from build123d import *

# Parameters (mm, degrees)
BOSS_EXTRUDE1_DEPTH = 17
BOSS_EXTRUDE2_DEPTH = 1.5
SKETCH3_R           = 1.45
CUT_EXTRUDE1_DEPTH  = 45.735332792
FILLET1_R           = 10
SKETCH4_R           = 5
CUT_EXTRUDE4_DEPTH  = 2
FILLET2_R           = 0.5
SKETCH5_W           = 31
SKETCH5_H           = 3
BOSS_EXTRUDE3_DEPTH = 30
SKETCH6_W           = 3
SKETCH6_H           = 3
BOSS_EXTRUDE4_DEPTH = 10
CHAMFER1_SIZE2      = 10
CHAMFER1_SIZE       = 2.679491924
FILLET3_R           = 5
FILLET4_R           = 2


# Some blends are built 0.0001 mm under size
with BuildPart() as part:
    # Sketch1 → Boss-Extrude1 (new, symmetric)
    with BuildSketch(Plane(origin=(0, 0, 0), x_dir=(1, 0, 0), z_dir=(0, 1, 0))):
        Polygon((15.5, 0), (-15.5, 0), (-15.5, 30), (-18.5, 30), (-18.5, -3), (-28.5, -3), (-28.5, -6), (28.5, -6), (28.5, -3), (18.5, -3), (18.5, 30), (15.5, 30), align=None)
    extrude(amount=BOSS_EXTRUDE1_DEPTH, both=True)

    # Sketch2 → Boss-Extrude2 (add, symmetric)
    with BuildSketch(Plane(origin=(0, 0, 0), x_dir=(1, 0, 0), z_dir=(0, 1, 0))):
        Polygon((18.5, 30), (18.5, -3), (28.5, -3), align=None)
    boss_extrude2 = extrude(amount=BOSS_EXTRUDE2_DEPTH, both=True)

    # Mirror1: Boss-Extrude2 across plane
    add(boss_extrude2.mirror(Plane(origin=(0, 0, 0), x_dir=(0, 0, 1), z_dir=(1, 0, 0))))

    # Sketch3 → Cut-Extrude1 (cut, through all)
    with BuildSketch(Plane(origin=(0, 0, 0), x_dir=(-1, 0, 0), z_dir=(0, 0, -1))):
        with Locations((0, -10.5)):
            Circle(SKETCH3_R)
    extrude(amount=-CUT_EXTRUDE1_DEPTH, mode=Mode.SUBTRACT)

    # Fillet1
    fillet1_edges = [part.edges().sort_by_distance(p)[0] for p in [
        (28.5, 17, 4.5),
        (-28.5, 17, 4.5),
    ]]
    fillet(fillet1_edges, radius=FILLET1_R)

    # Sketch4 → Cut-Extrude4 (cut)
    with BuildSketch(Plane(origin=(0, 0, 0), x_dir=(-1, 0, 0), z_dir=(0, 0, -1))):
        with Locations((0, -10.5)):
            Circle(SKETCH4_R)
    extrude(amount=-CUT_EXTRUDE4_DEPTH, mode=Mode.SUBTRACT)

    # Fillet2
    fillet2_edges = [part.edges().sort_by_distance(p)[0] for p in [
        (5, -10.5, 2),
    ]]
    fillet(fillet2_edges, radius=FILLET2_R)

    # Sketch5 → Boss-Extrude3 (add)
    with BuildSketch(Plane(origin=(0, 0, 0), x_dir=(-1, 0, 0), z_dir=(0, 0, -1))):
        with Locations((0, 15.5)):
            Rectangle(SKETCH5_W, SKETCH5_H)
    extrude(amount=BOSS_EXTRUDE3_DEPTH)

    # Sketch6 → Boss-Extrude4 (add)
    with BuildSketch(Plane(origin=(28.5, 0, 0), x_dir=(0, 0, -1), z_dir=(1, 0, 0))):
        with Locations((-4.5, -15.5)):
            Rectangle(SKETCH6_W, SKETCH6_H)
    extrude(amount=BOSS_EXTRUDE4_DEPTH)

    # Chamfer1
    chamfer1_edges = [part.edges().sort_by_distance(p)[0] for p in [
        (28.5, -14, 4.5),
    ]]
    chamfer1_side = [part.faces().sort_by_distance(p)[0] for p in [
        (28.5, -13.946410162, 4.5),
    ]]
    chamfer(chamfer1_edges, length=CHAMFER1_SIZE - 0.0001, length2=CHAMFER1_SIZE2 - 0.0001, reference=chamfer1_side[0])  # a hair under: the kernel refuses the full size

    # Fillet3
    fillet3_edges = [part.edges().sort_by_distance(p)[0] for p in [
        (18.5, 17, -13.5),
        (15.5, 14, -15),
        (-18.5, 17, -13.5),
        (-15.5, 14, -15),
    ]]
    fillet(fillet3_edges, radius=FILLET3_R)

    # Fillet4
    # the kernel refuses this fillet: 2 mm, written as the material it adds along each edge
    with BuildSketch(Plane(origin=(-20.5, 3.5, 1), x_dir=(0, 0, 1), z_dir=(1, 0, 0))) as fillet4_piece_1_section:
        Polygon((0, 0), (FILLET4_R * 1.02, 0), (FILLET4_R * 1.02, FILLET4_R * 1.02), (0, FILLET4_R * 1.02), align=None)
    fillet4_piece_1 = extrude(amount=FILLET4_R * 1.02, mode=Mode.PRIVATE)
    fillet4_piece_1 = fillet4_piece_1 - Plane(origin=(-20.5, 3.5, 1), x_dir=(0, 0.7071067811865475, -0.7071067811865475), z_dir=(1, 0, 0)) * Sphere(FILLET4_R, mode=Mode.PRIVATE)
    add(fillet4_piece_1)
    with BuildSketch(Plane(origin=(20.5, 3.5, 1), x_dir=(-1, 0, 0), z_dir=(0, 0, 1))) as fillet4_piece_2_section:
        Polygon((0, 0), (FILLET4_R * 1.02, 0), (FILLET4_R * 1.02, FILLET4_R * 1.02), (0, FILLET4_R * 1.02), align=None)
    fillet4_piece_2 = extrude(amount=FILLET4_R * 1.02, mode=Mode.PRIVATE)
    fillet4_piece_2 = fillet4_piece_2 - Plane(origin=(20.5, 3.5, 1), x_dir=(0.7071067811865475, 0.7071067811865475, 0), z_dir=(0, 0, 1)) * Sphere(FILLET4_R, mode=Mode.PRIVATE)
    add(fillet4_piece_2)
    with BuildSketch(Plane(origin=(20.5, -3.5, 1), x_dir=(-1, 0, 0), z_dir=(0, 1, 0))) as fillet4_piece_3_section:
        Polygon((0, 0), (FILLET4_R * 1.02, 0), (FILLET4_R * 1.02, FILLET4_R * 1.02), (0, FILLET4_R * 1.02), align=None)
    fillet4_piece_3 = extrude(amount=FILLET4_R * 1.02, mode=Mode.PRIVATE)
    fillet4_piece_3 = fillet4_piece_3 - Plane(origin=(20.5, -3.5, 1), x_dir=(0.7071067811865474, 0, -0.7071067811865477), z_dir=(0, 1, 0)) * Sphere(FILLET4_R, mode=Mode.PRIVATE)
    add(fillet4_piece_3)
    with BuildSketch(Plane(origin=(-20.5, -3.5, 1), x_dir=(0, 1, 0), z_dir=(0, 0, 1))) as fillet4_piece_4_section:
        Polygon((0, 0), (FILLET4_R * 1.02, 0), (FILLET4_R * 1.02, -FILLET4_R * 1.02), (0, -FILLET4_R * 1.02), align=None)
    fillet4_piece_4 = extrude(amount=FILLET4_R * 1.02, mode=Mode.PRIVATE)
    fillet4_piece_4 = fillet4_piece_4 - Plane(origin=(-20.5, -3.5, 1), x_dir=(-0.7071067811865475, -0.7071067811865475, 0), z_dir=(0, 0, 1)) * Sphere(FILLET4_R, mode=Mode.PRIVATE)
    add(fillet4_piece_4)
    with BuildSketch(Plane(origin=(28.5, -11.320608076, 3), x_dir=(0, 1, 0), z_dir=(0, 0, 1))) as fillet4_piece_5:
        with BuildLine():
            CenterArc((FILLET4_R * 0.767332413902, -FILLET4_R), FILLET4_R, 90, 75.000391344)
            Line((-FILLET4_R * 0.19859518016, -FILLET4_R * 0.741187552406), (0, 0))
            Line((0, 0), (FILLET4_R * 0.767332413902, 0))
        make_face()
    extrude(amount=3)
    with BuildSketch(Plane(origin=(-18.5, 3.5, 3), x_dir=(-1, 0, 0), z_dir=(0, 1, 0))) as fillet4_piece_6:
        with BuildLine():
            CenterArc((FILLET4_R, -FILLET4_R), FILLET4_R, 90, 90)
            Line((0, -FILLET4_R), (0, 0))
            Line((0, 0), (FILLET4_R, 0))
        make_face()
    extrude(amount=8.5)
    with BuildSketch(Plane(origin=(18.5, 3.5, 3), x_dir=(1, 0, 0), z_dir=(0, 1, 0))) as fillet4_piece_7:
        with BuildLine():
            CenterArc((FILLET4_R, FILLET4_R), FILLET4_R, 180, 90)
            Line((0, FILLET4_R), (0, 0))
            Line((0, 0), (FILLET4_R, 0))
        make_face()
    extrude(amount=8.5)
    with BuildSketch(Plane(origin=(-13.5, 12, 3), x_dir=(0.8416879607506226, 0.5399642365263262, 0), z_dir=(0.5399642365263262, -0.8416879607506226, 0))) as fillet4_piece_8_section:
        with BuildLine():
            CenterArc((5 + FILLET4_R, -FILLET4_R), FILLET4_R, 90, 90)
            Line((5 + FILLET4_R, 0), (5, 0))
            Line((5, 0), (5, -FILLET4_R))
        make_face()
    fillet4_piece_8 = revolve(axis=Axis((-13.5, 12, 3), (0, 0, 1)), revolution_arc=147.318795695, mode=Mode.PRIVATE)
    fillet4_piece_8 = split(fillet4_piece_8, bisect_by=Plane(origin=(-17.113068515, 17, 2.473069622), z_dir=(0, -1, 0)), keep=Keep.TOP, mode=Mode.PRIVATE)
    add(fillet4_piece_8)
    with BuildSketch(Plane(origin=(13.5, 12, 3), x_dir=(-0.8416879607506225, 0.5399642365263265, 0), z_dir=(-0.5399642365263265, -0.8416879607506225, 0))) as fillet4_piece_9_section:
        with BuildLine():
            CenterArc((5 + FILLET4_R, FILLET4_R), FILLET4_R, 180, 90)
            Line((5, FILLET4_R), (5, 0))
            Line((5, 0), (5 + FILLET4_R, 0))
        make_face()
    fillet4_piece_9 = revolve(axis=Axis((13.5, 12, 3), (0, 0, -1)), revolution_arc=147.318795695, mode=Mode.PRIVATE)
    fillet4_piece_9 = split(fillet4_piece_9, bisect_by=Plane(origin=(17.113068943, 17, 2.473070036), z_dir=(0, -1, 0)), keep=Keep.TOP, mode=Mode.PRIVATE)
    add(fillet4_piece_9)
    with BuildSketch(Plane(origin=(18.5, -17, 3), x_dir=(1, 0, 0), z_dir=(0, 1, 0)), Plane(origin=(-18.5, -17, 3), x_dir=(0, 0, -1), z_dir=(0, 1, 0))) as fillet4_piece_10:
        with BuildLine():
            CenterArc((FILLET4_R, FILLET4_R), FILLET4_R, 180, 90)
            Line((0, FILLET4_R), (0, 0))
            Line((0, 0), (FILLET4_R, 0))
        make_face()
    extrude(amount=13.5)
    with BuildSketch(Plane(origin=(18.5, -1.5, -35), x_dir=(0, -1, 0), z_dir=(0, 0, 1))) as fillet4_piece_11_section:
        with BuildLine():
            CenterArc((FILLET4_R, FILLET4_R), FILLET4_R, 180, 90)
            Line((0, FILLET4_R), (0, 0))
            Line((0, 0), (FILLET4_R, 0))
        make_face()
    fillet4_piece_11 = extrude(amount=36, mode=Mode.PRIVATE)
    fillet4_piece_11 = split(fillet4_piece_11, bisect_by=Plane(origin=(23.03556841, -1.955982706, -15.032624248), z_dir=(-0.9570244044334735, 0, 0.290007395282871)), keep=Keep.TOP, mode=Mode.PRIVATE)
    add(fillet4_piece_11)
    with BuildSketch(Plane(origin=(20.5, -1.5, 3), x_dir=(0, -1, 0), z_dir=(1, 0, 0))) as fillet4_piece_12_section:
        with BuildLine():
            CenterArc((FILLET4_R, FILLET4_R), FILLET4_R, 180, 90)
            Line((0, FILLET4_R), (0, 0))
            Line((0, 0), (FILLET4_R, 0))
        make_face()
    fillet4_piece_12 = extrude(amount=13, mode=Mode.PRIVATE)
    fillet4_piece_12 = split(fillet4_piece_12, bisect_by=Plane(origin=(28.035474122, -1.949923656, 1.467064601), z_dir=(-0.9570244044334735, 0, 0.290007395282871)), keep=Keep.TOP, mode=Mode.PRIVATE)
    add(fillet4_piece_12)
    with BuildSketch(Plane(origin=(18.5, 1.5, -35), x_dir=(0, 1, 0), z_dir=(0, 0, 1))) as fillet4_piece_13_section:
        with BuildLine():
            CenterArc((FILLET4_R, -FILLET4_R), FILLET4_R, 90, 90)
            Line((0, -FILLET4_R), (0, 0))
            Line((0, 0), (FILLET4_R, 0))
        make_face()
    fillet4_piece_13 = extrude(amount=36, mode=Mode.PRIVATE)
    fillet4_piece_13 = split(fillet4_piece_13, bisect_by=Plane(origin=(23.03556841, 1.955982706, -15.032624248), z_dir=(-0.9570244044334735, 0, 0.290007395282871)), keep=Keep.TOP, mode=Mode.PRIVATE)
    add(fillet4_piece_13)
    with BuildSketch(Plane(origin=(20.5, 1.5, 3), x_dir=(0, 1, 0), z_dir=(1, 0, 0))) as fillet4_piece_14_section:
        with BuildLine():
            CenterArc((FILLET4_R, -FILLET4_R), FILLET4_R, 90, 90)
            Line((0, -FILLET4_R), (0, 0))
            Line((0, 0), (FILLET4_R, 0))
        make_face()
    fillet4_piece_14 = extrude(amount=13, mode=Mode.PRIVATE)
    fillet4_piece_14 = split(fillet4_piece_14, bisect_by=Plane(origin=(28.035474122, 1.949923656, 1.467064601), z_dir=(-0.9570244044334735, 0, 0.290007395282871)), keep=Keep.TOP, mode=Mode.PRIVATE)
    add(fillet4_piece_14)
    with BuildSketch(Plane(origin=(-20.5, 1.5, 3), x_dir=(0, 1, 0), z_dir=(-1, 0, 0))) as fillet4_piece_15_section:
        with BuildLine():
            CenterArc((FILLET4_R, FILLET4_R), FILLET4_R, 180, 90)
            Line((0, FILLET4_R), (0, 0))
            Line((0, 0), (FILLET4_R, 0))
        make_face()
    fillet4_piece_15 = extrude(amount=13, mode=Mode.PRIVATE)
    fillet4_piece_15 = split(fillet4_piece_15, bisect_by=Plane(origin=(-28.035474122, 1.949923656, 1.467064601), z_dir=(0.9570244044334735, 0, 0.290007395282871)), keep=Keep.TOP, mode=Mode.PRIVATE)
    add(fillet4_piece_15)
    with BuildSketch(Plane(origin=(-18.5, 1.5, -35), x_dir=(0, 1, 0), z_dir=(0, 0, 1))) as fillet4_piece_16_section:
        with BuildLine():
            CenterArc((FILLET4_R, FILLET4_R), FILLET4_R, 180, 90)
            Line((0, FILLET4_R), (0, 0))
            Line((0, 0), (FILLET4_R, 0))
        make_face()
    fillet4_piece_16 = extrude(amount=36, mode=Mode.PRIVATE)
    fillet4_piece_16 = split(fillet4_piece_16, bisect_by=Plane(origin=(-23.03556841, 1.955982706, -15.032624248), z_dir=(0.9570244044334735, 0, 0.290007395282871)), keep=Keep.TOP, mode=Mode.PRIVATE)
    add(fillet4_piece_16)
    with BuildSketch(Plane(origin=(-18.5, -1.5, -35), x_dir=(0, -1, 0), z_dir=(0, 0, 1))) as fillet4_piece_17_section:
        with BuildLine():
            CenterArc((FILLET4_R, -FILLET4_R), FILLET4_R, 90, 90)
            Line((0, -FILLET4_R), (0, 0))
            Line((0, 0), (FILLET4_R, 0))
        make_face()
    fillet4_piece_17 = extrude(amount=36, mode=Mode.PRIVATE)
    fillet4_piece_17 = split(fillet4_piece_17, bisect_by=Plane(origin=(-23.03556841, -1.955982706, -15.032624248), z_dir=(0.9570244044334735, 0, 0.290007395282871)), keep=Keep.TOP, mode=Mode.PRIVATE)
    add(fillet4_piece_17)
    with BuildSketch(Plane(origin=(-20.5, -1.5, 3), x_dir=(0, -1, 0), z_dir=(-1, 0, 0))) as fillet4_piece_18_section:
        with BuildLine():
            CenterArc((FILLET4_R, -FILLET4_R), FILLET4_R, 90, 90)
            Line((0, -FILLET4_R), (0, 0))
            Line((0, 0), (FILLET4_R, 0))
        make_face()
    fillet4_piece_18 = extrude(amount=13, mode=Mode.PRIVATE)
    fillet4_piece_18 = split(fillet4_piece_18, bisect_by=Plane(origin=(-28.035474122, -1.949923656, 1.467064601), z_dir=(0.9570244044334735, 0, 0.290007395282871)), keep=Keep.TOP, mode=Mode.PRIVATE)
    add(fillet4_piece_18)


solid = part.part
Part model, mm, in its own coordinate system. A direction names the side the tool comes from. Give positions to 0.01 mm unless a question says otherwise; leave off trailing zeros. Order: outer loops, then holes, each group sorted by start corner. A loop starts at its lowest first (then second) coordinate and runs counter-clockwise, first axis right, second up. Notation, with made-up numbers: (-25, -10.5) - (15, -10.5) arc R12 ccw to (15, -5.5) - close; hole circle Ø9 at (80.5, -23). An arc over 180 degrees is marked (long way). Use a Markdown table: item, result.
1) Flat gauge pins, fed straight in: P1, Ø8, axis at y = 0.5, z = -19.5, coming from the +X side; P2, Ø8, axis at x = -23.5, z = -15.5, coming from the -Y side; P3, Ø1, axis at x = 2.5, y = -7, coming from the -Z side. Where does each tip first touch, or does it go through?
Checked values:
| item | result |
|---|---|
| P1 | x = 22.89 |
| P2 | y = -1.77 |
| P3 | z = 1.9 |
2) Saw through at A-A on x = 0. List the corners of the cut face in (y, z), plus the area to 3 significant figures.
Checked values:
| item | result |
|---|---|
| outline | (-17, 0) - (-15.5, 0) - (-15.5, 1.5) arc R0.5 cw to (-15, 2) - (-11.95, 2) - (-11.95, 6) - (-17, 6) - close; (-9.05, 2) - (-6, 2) arc R0.5 cw to (-5.5, 1.5) - (-5.5, 0) - (14, 0) - (14, -30) - (17, -30) - (17, 6) - (-9.05, 6) - close |
| area | 263 mm² |
3) 3-axis set-ups, long thin cutter, end or side, ignore diameter. For faces 1 (the flat face through (18.5, 8, -14)), 2 (the cylindrical face through (14.07, 12.5, -15.21)), 3 (the cylindrical face through (-19.07, -2.1, -14.72)), 4 (the cylindrical face through (-19.1, 2.07, -14.72)): which of +Z, -Z, +X, -X, +Y, -Y reach the whole face in a straight line?
Checked values:
| item | result |
|---|---|
| face 1 | -Z, +X, +Y |
| face 2 | -Z, -Y |
| face 3 | -Z, -X, -Y |
| face 4 | -Z, -X, +Y |
4) Saw through at B-B on y = -10.5. List the corners of the cut face in (x, z), plus the area to 3 significant figures.
Checked values:
| item | result |
|---|---|
| outline | (-28.5, 3) - (-20.5, 3) arc R2 cw to (-18.5, 1) - (-18.5, -30) - (-15.5, -30) - (-15.5, 0) - (-5, 0) - (-5, 1.5) arc R0.5 cw to (-4.5, 2) - (-1.45, 2) - (-1.45, 6) - (-28.5, 6) - close; (1.45, 2) - (4.5, 2) arc R0.5 cw to (5, 1.5) - (5, 0) - (15.5, 0) - (15.5, -30) - (18.5, -30) - (18.5, 1) arc R2 cw to (20.5, 3) - (28.63, 3) - (28.63, 6) - (1.45, 6) - close |
| area | 433 mm² |
5) Saw through at D-D on x = 12. List the corners of the cut face in (y, z).
Checked values:
| item | result |
|---|---|
| outline | (-17, 0) - (13.77, 0) - (13.77, -30) - (17, -30) - (17, 6) - (-17, 6) - close |
6) Saw through at C-C on z = -18. List the corners of the cut face in (x, y), plus the area to 3 significant figures.
Checked values:
| item | result |
|---|---|
| outline | (-22.14, -1.5) - (-20.5, -1.5) arc R2 cw to (-18.5, -3.5) - (-18.5, -17) - (-15.5, -17) - (-15.5, 9) arc R5 cw to (-10.5, 14) - (10.5, 14) arc R5 cw to (15.5, 9) - (15.5, -17) - (18.5, -17) - (18.5, -3.5) arc R2 cw to (20.5, -1.5) - (22.14, -1.5) - (22.14, 1.5) - (20.5, 1.5) arc R2 cw to (18.5, 3.5) - (18.5, 12) arc R5 ccw to (13.5, 17) - (-13.5, 17) arc R5 ccw to (-18.5, 12) - (-18.5, 3.5) arc R2 cw to (-20.5, 1.5) - (-22.14, 1.5) - close |
| area | 322 mm² |
7) Probe L1, parallel to Y at x = 0, z = 5.2; L2, parallel to Y at x = 0, z = 0.65; L3, parallel to X at y = -9.5, z = -24. List the from-to ranges inside material, lowest first. Write a range as from..to.
Checked values:
| item | result |
|---|---|
| L1 | -17..-11.95, -9.05..17 |
| L2 | -17..-15.5, -5.5..17 |
| L3 | -18.5..-15.5, 15.5..18.5 |
8) Two-plate mould, pull along X, no slides. Class faces 5 (the flat face through (-15.5, -4, -15)), 6 (the flat face through (24, 9, 3)), 7 (the cylindrical face through (28.902, -10.989, 4.479)), 8 (the flat face through (-18.5, 8, -15)): +X half, -X half, draft (parallel to the pull), parting line (faces both ways), or undercut.
Checked values:
| item | result |
|---|---|
| face 5 | undercut |
| face 6 | draft |
| face 7 | +X half |
| face 8 | -X half |
